Input: part model. Units: mm. Frame: model coordinates. Give positions to 0.01 mm unless a question says otherwise; leave off trailing zeros. Write each loop counter-clockwise with the first axis right and the second up, starting at its lowest first coordinate (ties: lowest second). Pieces come first, ordered by that corner, then holes. Notation, with made-up numbers: (56, 32) -> (69, 32) arc R10 ccw to (69, 42) -> close; hole circle Ø1 at (68.5, 17.5). An arc over 180 degrees is marked (long way). Return JSON: item names as keys, results as strings. Group by question number.
Item 1: Line query: line 1 (Z direction, x = 0, y = 2.4); line 2 (Y direction, x = 25.5, z = 24.5). Output: solid intervals per line, ascending. Write a range as [from, to].
Item 2: Section D-D, the plane x = -29.25. Return loops of the section in (y, z), then the cut area to 3 significant figures.
Item 3: Pin query (flat end, axial travel): P1, Ø1, axis at y = 3, z = -13, coming from the -X side; P2, Ø2, axis at x = -4, z = 19.5, coming from the -Y side; P3, Ø1.5, axis at x = 15, z = 26, coming from the +Y side. Return the tip coordinate at first contact, or that it passes through.
Item 4: Section B-B, the plane z = 5.5. Return loops of the section in (x, y).
Item 5: Section A-A, the plane x = 0. Return loops of the section in (y, z), then the cut area to 4 significant figures.
Item 6: Section C-C, the plane y = 5.8. Return loops of the section in (x, z).
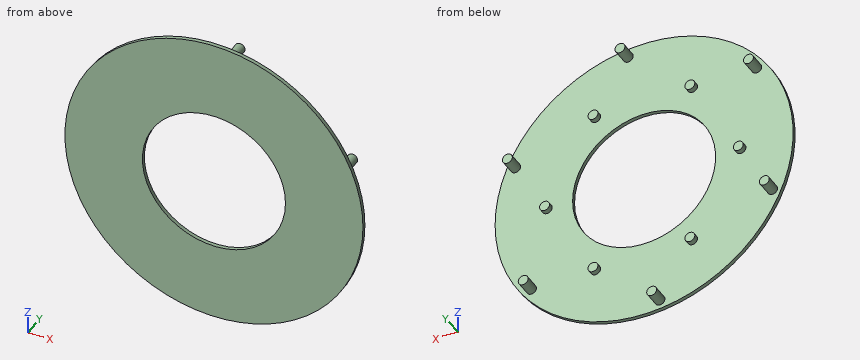
from build123d import *

# Parameters (mm, degrees)
SKETCH1_R           = 200
SKETCH1_R_2         = 96
BOSS_EXTRUDE1_DEPTH = 5
SKETCH2_R           = 3.5
SKETCH2_R_2         = 2
CUT_EXTRUDE1_DEPTH  = 5
CIRPATTERN1_COUNT   = 6
SCALE2_SCALE        = 0.225
SKETCH3_R           = 1.5
BOSS_EXTRUDE2_DEPTH = 5.93
SKETCH4_R           = 1.5
BOSS_EXTRUDE3_DEPTH = 2.7
CIRPATTERN2_COUNT   = 6


with BuildPart() as part:
    # Sketch1 → Boss-Extrude1 (new body)
    with BuildSketch(Plane(origin=(0, 0, 0), x_dir=(1, 0, 0), z_dir=(0, 1, 0))):
        Circle(SKETCH1_R)
        Circle(SKETCH1_R_2, mode=Mode.SUBTRACT)
    extrude(amount=BOSS_EXTRUDE1_DEPTH)

    # Sketch2 → Cut-Extrude1 (cut)
    with BuildSketch(Plane(origin=(0, 5, 0), x_dir=(1, 0, 0), z_dir=(0, 1, 0))):
        with Locations((151.125089796, 111.826683909)):
            Circle(SKETCH2_R)
        with Locations((130, 0)):
            Circle(SKETCH2_R_2)
    cut_extrude1 = extrude(amount=-CUT_EXTRUDE1_DEPTH, mode=Mode.SUBTRACT)

    # CirPattern1: Cut-Extrude1 ×6 about axis
    cirpattern1_axis = Axis((0, 0, 0), (0, 1, 0))
    for i in range(1, CIRPATTERN1_COUNT):
        add(cut_extrude1.rotate(cirpattern1_axis, i * 360 / CIRPATTERN1_COUNT), mode=Mode.SUBTRACT)


with BuildPart() as part_1:
    # Scale2: scaled about (0, 2.5, 0)
    add(part.part.scale(SCALE2_SCALE).moved(Location((0, 1.9375, 0))))

    # Sketch3 → Boss-Extrude2 (add)
    with BuildSketch(Plane.XZ.offset(-1.9375)):
        with Locations((-38.791641146, -16.867085616)):
            Circle(SKETCH3_R)
    boss_extrude2 = extrude(amount=-BOSS_EXTRUDE2_DEPTH)

    # Sketch4 → Boss-Extrude3 (add)
    with BuildSketch(Plane.XZ.offset(-1.9375)):
        with Locations((-14.625, 25.331243061)):
            Circle(SKETCH4_R)
        with Locations((14.625, 25.331243061)):
            Circle(SKETCH4_R)
        with Locations((29.25, 0)):
            Circle(SKETCH4_R)
        with Locations((14.625, -25.331243061)):
            Circle(SKETCH4_R)
        with Locations((-14.625, -25.331243061)):
            Circle(SKETCH4_R)
        with Locations((-29.25, 0)):
            Circle(SKETCH4_R)
    extrude(amount=-BOSS_EXTRUDE3_DEPTH)

    # CirPattern2: Boss-Extrude2 ×6 about axis
    cirpattern2_axis = Axis((0, 0, 0), (0, 1, 0))
    for i in range(1, CIRPATTERN2_COUNT):
        add(boss_extrude2.rotate(cirpattern2_axis, i * 360 / CIRPATTERN2_COUNT))


solid = part_1.part
Answer below:
{
 "1": {"line 1": "z = [-45, -21.6], [21.6, 45]", "line 2": "y = [1.94, 3.06]"},
 "2": {"outline": "(1.94, -34.2) -> (3.06, -34.2) -> (3.06, -1.5) -> (4.64, -1.5) -> (4.64, 1.5) -> (3.06, 1.5) -> (3.06, 34.2) -> (1.94, 34.2) -> close", "area": "81.7 mm2"},
 "3": {"P1": "stops at x = -43.23", "P2": "passes through", "P3": "stops at y = 4.64"},
 "4": {"outline": "(-44.66, 1.94) -> (-20.89, 1.94) -> (-20.89, 3.06) -> (-44.66, 3.06) -> close; (20.89, 1.94) -> (44.66, 1.94) -> (44.66, 3.06) -> (20.89, 3.06) -> close"},
 "5": {"outline": "(1.94, -45) -> (3.06, -45) -> (3.06, -21.6) -> (1.94, -21.6) -> close; (1.94, 21.6) -> (3.06, 21.6) -> (3.06, 45) -> (1.94, 45) -> close", "area": "52.65 mm2"},
 "6": {"outline": "circle Ø3 at (-38.79, -16.87); circle Ø3 at (-34, 25.16); circle Ø3 at (-4.79, -42.03); circle Ø3 at (4.79, 42.03); circle Ø3 at (34, -25.16); circle Ø3 at (38.79, 16.87)"}
}
